The listing builds one solid part. Answer for the finished solid, in the listing's coordinates (mm). A direction names the side the tool comes from. Coordinates: 2 decimals unless noted, no trailing zeros. Write each loop counter-clockwise with the first axis right and the second up, starting at its lowest first coordinate (ties: lowest second). Pieces come first, ordered by that corner, then holes.
```python
from build123d import *

# Parameters (mm, degrees)
F1_DEPTH = 2000


with BuildPart() as f1:
    # F0 (on Front) → F1 (new body)
    with BuildSketch(Plane.XZ):
        with BuildLine():
            Line((-25, 0), (0, 0))
            Line((0, 0), (25, 0))
            ThreePointArc((25, 0), (28.535534, 1.464466), (30, 5))
            Line((30, 5), (30, 46))
            Line((30, 46), (27, 50))
            Line((27, 50), (27.798945, 51.864205))
            ThreePointArc((27.798945, 51.864205), (28.000636, 52.22595), (28.272511, 52.538396))
            ThreePointArc((28.272511, 52.538396), (29.647293, 54.571329), (30, 57))
            ThreePointArc((30, 57), (22.611278, 59.631425), (19.08164, 52.627194))
            Line((19.08164, 52.627194), (21.016316, 53.134174))
            ThreePointArc((21.016316, 53.134174), (23.152059, 57.686868), (28.01478, 56.405318))
            ThreePointArc((28.01478, 56.405318), (27.697789, 55.094007), (26.907788, 54.000425))
            ThreePointArc((26.907788, 54.000425), (26.364036, 53.375534), (25.960655, 52.652043))
            Line((25.960655, 52.652043), (25.16171, 50.787839))
            Line((25.16171, 50.787839), (24.706223, 49.725036))
            Line((24.706223, 49.725036), (28, 45.333333))
            Line((28, 45.333333), (28, 5))
            ThreePointArc((28, 5), (27.12132, 2.87868), (25, 2))
            Line((25, 2), (0, 2))
            Line((0, 2), (-25, 2))
            ThreePointArc((-25, 2), (-27.12132, 2.87868), (-28, 5))
            Line((-28, 5), (-28, 45.333333))
            Line((-28, 45.333333), (-24.706223, 49.725036))
            Line((-24.706223, 49.725036), (-25.16171, 50.787839))
            Line((-25.16171, 50.787839), (-25.960655, 52.652043))
            ThreePointArc((-25.960655, 52.652043), (-26.364036, 53.375534), (-26.907788, 54.000425))
            ThreePointArc((-26.907788, 54.000425), (-27.697789, 55.094007), (-28.01478, 56.405318))
            ThreePointArc((-28.01478, 56.405318), (-23.152059, 57.686868), (-21.016316, 53.134174))
            Line((-21.016316, 53.134174), (-19.08164, 52.627194))
            ThreePointArc((-19.08164, 52.627194), (-22.611278, 59.631425), (-30, 57))
            ThreePointArc((-30, 57), (-29.647293, 54.571329), (-28.272511, 52.538396))
            ThreePointArc((-28.272511, 52.538396), (-28.000636, 52.22595), (-27.798945, 51.864205))
            Line((-27.798945, 51.864205), (-27, 50))
            Line((-27, 50), (-30, 46))
            Line((-30, 46), (-30, 5))
            ThreePointArc((-30, 5), (-28.535534, 1.464466), (-25, 0))
        make_face()
    extrude(amount=-F1_DEPTH)


solid = f1.part
```
(1) For a pull along Z with two mould halves and no side action, classify faces 1 (the flat face through (0, 0, 1)), 2 (the flat face through (0, 986, 2)), 3 (the flat face through (0, 986, 0)) as pulls with the +Z half, pulls with the -Z half, needs draft (parallel to the pull), parting line crosses it, or undercut.
(2) Section C-C, the plane x = -9.5 is taken. Write down the section's boundary in (y, z), plus the area to 3 significant figures.
(3) Each of these flat-tipped pins is pushed along its axis until it touches: pin 1 (12 mm diameter, centred on y = 1356, z = 16.5, fed in from +X); pin 2 (1.5 mm diameter, centred on x = 11.5, y = 624.5, fed in from +Z); pin 3 (3 mm diameter, centred on x = 19.5, y = 1320.5, fed in from +Z). Where does it stop, or does it pass through?
(4) Find the intervals of material crossed by probe 1 along Z at (x, y) = (25, 1769); probe 2 along X at (y, z) = (478.5, 52); probe 3 along X at (y, z) = (1236.5, 56), in increasing order.
(5) Which of the six approach directions +Z, -Z, +X, -X, +Y, -Y give full straight-line access (tool end or side, diameter ignored) to faces 4 (the flat face through (28, 986, 25)), 5 (the flat face through (30, 986, 25))?
(6) Section A-A, the plane z = 33 is taken. Write down the section's boundary in (x, y).
Solution:
1. face 1: needs draft
1. face 2: undercut
1. face 3: pulls with the -Z half
2. outline: (0, 0) - (2000, 0) - (2000, 2) - (0, 2) - close
2. area: 4,000 mm2
3. pin 1: stops at x = 30
3. pin 2: stops at z = 2
3. pin 3: stops at z = 58.67
4. probe 1: z = 0 to 2, 49.33 to 50.41, 58.05 to 60.05
4. probe 2: x = -27.86 to -25.68, 25.68 to 27.86
4. probe 3: x = -29.99 to -27.97, -21.36 to -19.19, 19.19 to 21.36, 27.97 to 29.99
5. face 4: +Y, -Y
5. face 5: +Z, -Z, +X, +Y, -Y
6. outline: (-30, 0) - (-28, 0) - (-28, 2000) - (-30, 2000) - close; (28, 0) - (30, 0) - (30, 2000) - (28, 2000) - close
